Can you work these out from the model? Positions are in its coordinate system, mm. Face numbers are marked on the shaded views. A direction names the side the tool comes from. Coordinates: 2 decimals unless noted, no trailing zeros. Loops run counter-clockwise (first coordinate to the right, second up) from the corner with the lowest first, then second, coordinate; pieces in that order, holes last. Notation, with made-up numbers: M 66,9 L 112,9 A20 ccw 112,19 Z; hole C 17,-27.75 d10. An arc over 180 degrees is marked long. Return JSON: item names as keys, results as strings. Group by question number.
```python
from build123d import *

# Parameters (mm, degrees)
F0_R          = 4
F0_R_2        = 2
F1_DEPTH      = 34
F2_DEPTH      = 46
F4_SIZE       = 0.5
F6_D          = 3.2
F6_DEPTH      = 14
F6_TIP        = 0.9613769904
F8_DEPTH      = 2
F7_W          = 8
F7_H          = 1.5
F9_DEPTH      = 10
F9_DEPTH_BACK = 2
F10_R         = 1.6
F11_DEPTH     = 2.501


with BuildPart() as f1:
    # F0 (on Front) → F1 (new body)
    with BuildSketch(Plane.XZ):
        Circle(F0_R)
        Circle(F0_R_2, mode=Mode.SUBTRACT)
        Circle(F0_R_2)
    extrude(amount=F1_DEPTH)

    # F0 (on Front) → F2 (join)
    with BuildSketch(Plane.XZ):
        Circle(F0_R_2)
    extrude(amount=F2_DEPTH)

    # F4
    f4_edges = [f1.edges().sort_by_distance(p)[0] for p in [
        (-2, -46, 0),
    ]]
    chamfer(f4_edges, length=F4_SIZE)

    # F6
    with Locations(Plane(origin=(0, 0, 0), x_dir=(-1, 0, 0), z_dir=(0, 1, 0))):
        with Locations((0, 0)):
            Hole(F6_D / 2, depth=F6_DEPTH)
            with Locations((0, 0, -(F6_DEPTH + F6_TIP / 2))):  # 118° drill point
                Cone(0, F6_D / 2, F6_TIP, mode=Mode.SUBTRACT)

    # F7 (on offset) → F8 (cut, symmetric)
    with BuildSketch(Plane.XZ.offset(11.5)):
        Polygon((-3.7080992435, 4), (-3.7080992435, 1.5), (-2.1, 2.5), (2.1, 2.5), (3.7080992435, 1.5), (3.7080992435, 4), align=None)
    extrude(amount=F8_DEPTH, both=True, mode=Mode.SUBTRACT)

    # F7 (on offset) → F9 (cut, two sides)
    with BuildSketch(Plane.XZ.offset(11.5)) as f9_sk:
        with Locations((0, -3.25)):
            Rectangle(F7_W, F7_H)
    extrude(amount=F9_DEPTH, mode=Mode.SUBTRACT)
    extrude(f9_sk.sketch, amount=-F9_DEPTH_BACK, mode=Mode.SUBTRACT)

    # F10 (on face) → F11 (cut, through all)
    with BuildSketch(Plane.XY.offset(2.5)):
        with Locations((0, -11.5)):
            Circle(F10_R)
    extrude(amount=-F11_DEPTH, mode=Mode.SUBTRACT)


solid = f1.part
```
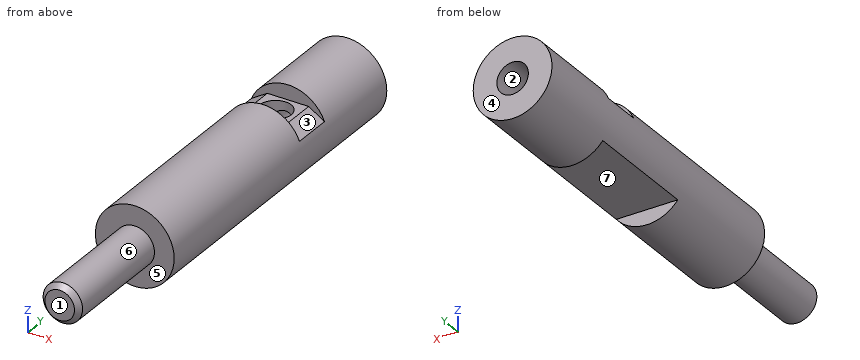
1) Suppose I cut it at B-B, the plane z = 3. List the corners of the cut face in (x, y) for me.
2) Suppose I cut it at A-A, the plane y = -11.5. List the corners of the cut face in (x, z) for me, then the cut area to 3 significant figures.
3) For the marked faces 1, 2 and 3, which set-ups out of +Z, -Z, +X, -X, +Y, -Y let a thin tool reach every point of the face, with its end or its side?
4) If I drill on line 1 (X direction, y = -10.5, z = -1); line 2 (Y direction, x = -2, z = -2.25); line 3 (X direction, y = -11.5, z = 1.1), over which ranges is the centre line in solid material (lowest first)? Write a range as from..to.
5) For pin 1 (2 mm diameter, centred on x = -0.5, z = 3, fed in from -Y); pin 2 (1.9 mm diameter, centred on x = 0, y = -17.5, fed in from -Z); pin 3 (1.5 mm diameter, centred on x = 0.5, y = -38, fed in from -Z), each with a flat end and sliding along its axis, tell me the tip position at first contact or that it passes through.
6) If we mould it in two halves opening along Y, with no side actions, what happens to the marked faces 4, 5, 6 and 7? For each: +Y half, -Y half, draft (parallel to the pull), parting line (faces both ways), or undercut.
7) Suppose I cut it at C-C, the plane y = -40.5. List the corners of the cut face in (x, z) for me, then the cut area to 3 significant figures.
Returned:
{
 "1": {"outline": "M -2.65,-34 L 2.65,-34 L 2.65,-13.5 L -2.65,-13.5 Z; M -2.65,-9.5 L 2.65,-9.5 L 2.65,0 L -2.65,0 Z"},
 "2": {"outline": "M -3.71,1.5 A4 ccw -3.12,-2.5 L 3.12,-2.5 A4 ccw 3.71,1.5 L 2.1,2.5 L 1.6,2.5 L 1.6,0 A1.6 cw -1.6,0 L -1.6,2.5 L -2.1,2.5 Z", "area": "24.1 mm²"},
 "3": {"face 1": "+Z, -Z, +X, -X, -Y", "face 2": "+Y", "face 3": "+Z, +X"},
 "4": {"line 1": "x = -3.87..-1.25, 1.25..3.87", "line 2": "y = -34..0", "line 3": "x = -3.85..-1.6, 1.6..3.85"},
 "5": {"pin 1": "stops at y = -34", "pin 2": "stops at z = -2.5", "pin 3": "stops at z = -2"},
 "6": {"face 4": "+Y half", "face 5": "-Y half", "face 6": "draft", "face 7": "undercut"},
 "7": {"outline": "C 0,0 d4", "area": "12.6 mm²"}
}
